Can you work these out from the model? Positions are in its coordinate system, mm. Face numbers are marked on the shaded views. A direction names the side the tool comes from. Give positions to 0.01 mm unless a question says otherwise; leave off trailing zeros. Write each loop counter-clockwise with the first axis right and the second up, starting at its lowest first coordinate (ties: lowest second). Pieces come first, ordered by that corner, then holes. Notation, with made-up numbers: (60.5, 56) - (66.5, 56) arc R24 cw to (66.5, 66) - close; hole circle Ø1 at (-29.5, 36.25). An arc over 180 degrees is marked (long way). Return JSON: item names as keys, results as strings. Group by question number.
Autodesk Inventor part; units mm, degrees
ref_plane "YZ Plane" through (0, 0, 0) normal (1, 0, 0) x (0, 1, 0)
ref_plane "XZ Plane" through (0, 0, 0) normal (0, 1, 0) x (-1, 0, 0)
ref_plane "XY Plane" through (0, 0, 0) normal (0, 0, 1) x (1, 0, 0)
sketch "Sketch1" plane through (0, 0, 0) normal (0, 0, 1) x (1, 0, 0)
  arc A0 (3.5439, 9.7114) -> (3.9233, 13.2109) centre (1.7309, 11.6783) ccw
  line L0 (3.9233, 13.2109) -> (-0.0821, 13.6452)
  arc A1 (-0.0821, 13.6452) -> (-0.4616, 10.1457) centre (1.7309, 11.6783) ccw
  line L1 (-0.4616, 10.1457) -> (3.5439, 9.7114)
  circle A2 centre (1.7309, 11.6783) radius 1.04
  circle A3 centre (1.7309, 11.6783) radius 25
  line L2 (-0.1489, 13.8536) -> (4.0332, 13.4001)
  arc A4 (3.6107, 9.503) -> (4.0332, 13.4001) centre (1.7309, 11.6783) ccw
  line L3 (3.6107, 9.503) -> (-0.5715, 9.9564)
  arc A5 (-0.1489, 13.8536) -> (-0.5715, 9.9564) centre (1.7309, 11.6783) ccw
  point P0 (0, 0)
  dimension "d0" = 50
  dimension "d1" = 0.2
extrude "Extrusion1" add sketch "Sketch1" along normal blind 15 contours A3
sketch "Sketch2" plane through (1.7309, 11.6783, 0) normal (0, 0, -1) x (-1, 0, 0)
  arc A0 (-2.3024, 1.7218) -> (-1.8798, -2.1753) centre (0, 0) ccw
  circle A1 centre (0, 0) radius 25
  line L0 (-1.8798, -2.1753) -> (2.3024, -1.7218)
  arc A2 (-2.3024, 1.7218) -> (-1.8798, -2.1753) centre (0, 0) ccw
  line L1 (1.8798, 2.1753) -> (-2.3024, 1.7218)
  arc A3 (2.3024, -1.7218) -> (1.8798, 2.1753) centre (0, 0) ccw
  circle A4 centre (0, 0) radius 5
  circle A5 centre (0, 0) radius 25
  point P0 (1.7309, -11.6783)
  dimension "d4" = 10
extrude "Extrusion2" cut sketch "Sketch2" against normal blind 7.5 contours A1
properties part number "Wheel"
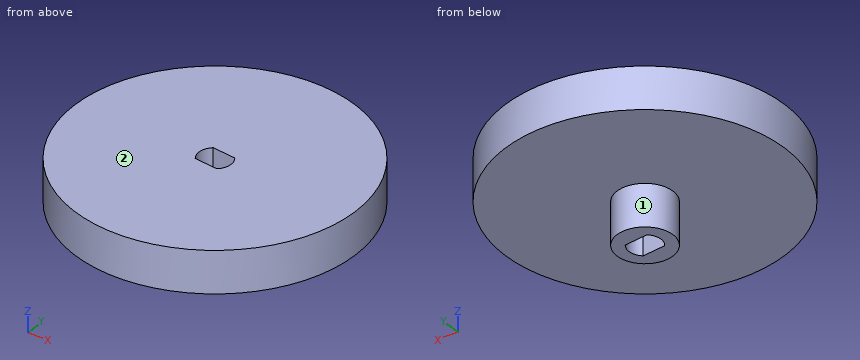
1) Will these pins go through, and if not, where does the flat tip stop? pin 1 Ø2 at (x, z) = (17.5, 12) entering from -Y; pin 2 Ø5 at (x, y) = (11, 27) entering from -Z; pin 3 Ø25 at (x, y) = (-9, 17.5) entering from -Z; pin 4 Ø4 at (x, z) = (-2, 7) entering from +Y.
2) Imagine slicing it at C-C, the plane y = 15. Write out the boundary of the cut face in (x, z).
3) On a 3-axis mill with a long thin cutter (end or side, diameter ignored), from which of +Z, -Z, +X, -X, +Y, -Y can I reach the whole of each face in a straight line? I mean the marked faces 1 and 2. Say none if no direction works.
4) I need wall thicknesses on line 1 along Z through (x, y) = (13, 23.5); line 2 along Y through (x, z) = (2, 7.25); line 3 along X through (y, z) = (12.5, 2.25). Which ranges of each line are inside material? Lowest first, please.
5) Imagine slicing it at A-A, the plane z = 4.25. Write out the boundary of the cut face in (x, y), and give its area (3 significant figures).
6) Imagine slicing it at D-D, the plane z = 10. Write out the boundary of the cut face in (x, y).
7) Imagine slicing it at B-B, the plane x = 5.5. Write out the boundary of the cut face in (y, z).
Resolved:
{
 "1": {"pin 1": "y = -8.49", "pin 2": "z = 7.5", "pin 3": "z = 0", "pin 4": "y = 36.61"},
 "2": {"outline": "(-23.05, 7.5) - (-2.01, 7.5) - (-2.01, 0) - (5.47, 0) - (5.47, 7.5) - (26.51, 7.5) - (26.51, 15) - (-23.05, 15) - close"},
 "3": {"face 1": "-Z", "face 2": "+Z, +X, -X, +Y, -Y"},
 "4": {"line 1": "7.5 to 15", "line 2": "6.69 to 9.68, 13.62 to 16.67", "line 3": "-3.2 to -1.02, 4.49 to 6.66"},
 "5": {"outline": "circle Ø10 at (1.73, 11.68); hole (-0.57, 9.96) - (3.61, 9.5) arc R2.87 ccw to (4.03, 13.4) - (-0.15, 13.85) arc R2.88 ccw to start", "area": "57.9 mm^2"},
 "6": {"outline": "circle Ø50 at (1.73, 11.68); hole (-0.57, 9.96) - (3.61, 9.5) arc R2.87 ccw to (4.03, 13.4) - (-0.15, 13.85) arc R2.88 ccw to start"},
 "7": {"outline": "(-13.04, 7.5) - (8.39, 7.5) - (8.39, 0) - (14.96, 0) - (14.96, 7.5) - (36.39, 7.5) - (36.39, 15) - (-13.04, 15) - close"}
}
